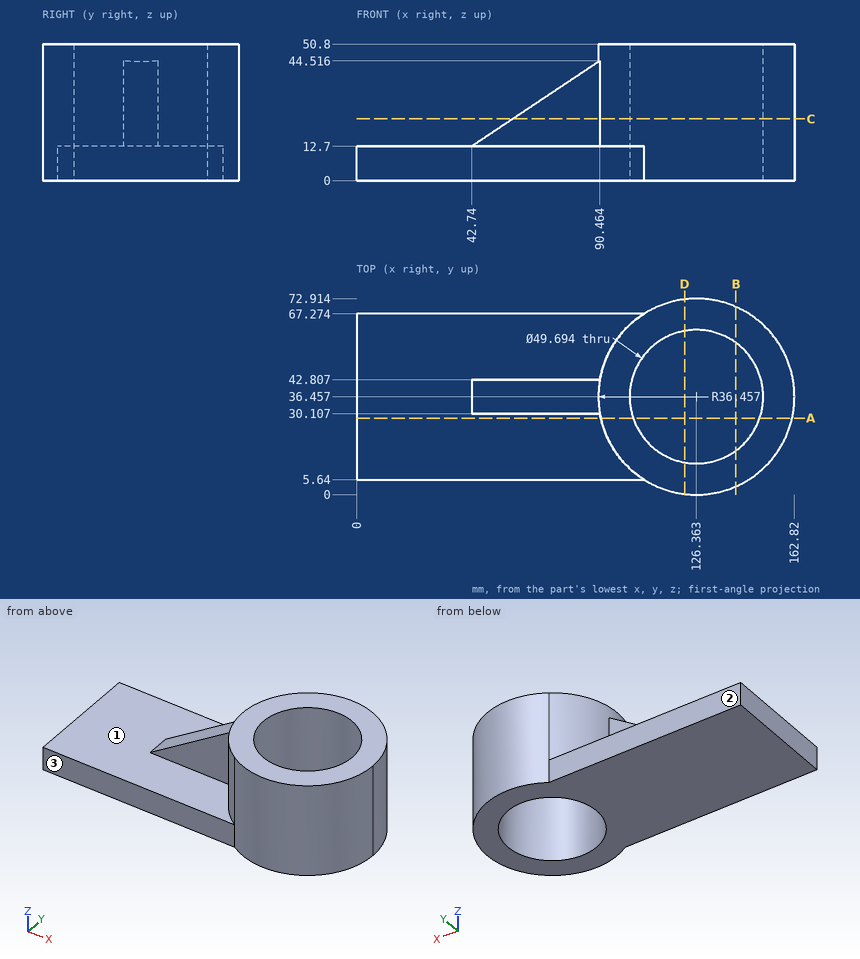
The figure shows three views and two pictorial views of one solid part (mm, origin at its lowest corner). Answer the questions. A direction names the side the tool comes from. Give positions to 0.01 mm unless a question says otherwise; leave off trailing zeros. Write each loop counter-clockwise with the first axis right and the second up, starting at its lowest first coordinate (ties: lowest second). Pieces come first, ordered by that corner, then holes. Notation, with made-up numbers: (-3, 30.5) - (12, 30.5) arc R31 cw to (12, 65.5) - close; hole circle Ø3 at (84, 61). An arc over 180 degrees is marked (long way). Use CSV: the item, a comma, the result in double quotes. Start each with the question number.
Item 1: The part is cut by section C-C, the plane z = 23. Give the vertices of the cut face in (x, y) (1 decimal), and give its area (3 significant figures).
Item 2: The part is cut by section B-B, the plane x = 141. Give the vertices of the cut face in (y, z) (1 decimal).
Item 3: The part is cut by section A-A, the plane y = 28.5. Give the vertices of the cut face in (x, z) (1 decimal), and give its area (3 significant figures).
Item 4: The part is cut by section D-D, the plane x = 122. Give the vertices of the cut face in (y, z) (1 decimal), and give its area (3 significant figures).
Item 5: For the marked faces 1, 2 and 3, determine the directions among +Z, -Z, +X, -X, +Y, -Y from which every point of the face is accessible in a straight line to the end or side of a thin tool.
Item 6: Flat-ended cylindrical pins translate along their axes: P1, Ø10, axis at x = 46, z = 3.5, coming from the +Y side; P2, Ø4, axis at y = 65, z = 36.5, coming from the +X side (1 decimal); P3, Ø2, axis at y = 51.5, z = 36, coming from the +X side; P4, Ø9.5, axis at x = 55, z = 31, coming from the -Y side. Find the tip coordinate at first contact, or state that the pin passes through.
Item 7: Consider line 1 (Z direction, x = 63, y = 25); line 2 (Y direction, x = 10.5, z = 7.5); line 3 (Y direction, x = 74.5, z = 33). Determine where each line is inside the solid, lowest interval first.
Taken from the geometry:
1,outline,"(58.2, 30.1) - (90.5, 30.1) arc R36.5 ccw to (106.9, 5.6) arc R36.5 ccw (long way) to (106.9, 67.3) arc R36.5 ccw to (90.5, 42.8) - (58.2, 42.8) - close; hole circle Ø49.7 at (126.4, 36.5)"
1,area,"2,640 mm2"
2,outline,"(3.1, 0) - (16.4, 0) - (16.4, 50.8) - (3.1, 50.8) - close; (56.5, 0) - (69.8, 0) - (69.8, 50.8) - (56.5, 50.8) - close"
3,outline,"(0, 0) - (102.8, 0) - (102.8, 50.8) - (90.8, 50.8) - (90.8, 12.7) - (0, 12.7) - close; (149.9, 0) - (161.9, 0) - (161.9, 50.8) - (149.9, 50.8) - close"
3,area,"2,380 mm2"
4,outline,"(0.3, 0) - (12, 0) - (12, 50.8) - (0.3, 50.8) - close; (60.9, 0) - (72.7, 0) - (72.7, 50.8) - (60.9, 50.8) - close"
4,area,"1,190 mm2"
5,face 1,"+Z, -X"
5,face 2,"+Z, -Z, -X, +Y"
5,face 3,"+Z, -Z, -X, -Y"
6,P1,"y = 67.27"
6,P2,"x = 151.4"
6,P3,"x = 160.01"
6,P4,"through"
7,line 1,"0 to 12.7"
7,line 2,"5.64 to 67.27"
7,line 3,"30.11 to 42.81"
